```python
from build123d import *

# Parameters (mm, degrees)
CROQUIS1_W              = 4
CROQUIS1_H              = 15
CROQUIS1_W_2            = 15
CROQUIS1_W_3            = 16
CROQUIS1_R              = 1.5
SALIENTE_EXTRUIR1_DEPTH = 4
CROQUIS2_W              = 4
CROQUIS2_H              = 15
SALIENTE_EXTRUIR2_DEPTH = 60
SALIENTE_EXTRUIR4_START = -7.5
SALIENTE_EXTRUIR4_DEPTH = 15
CROQUIS8_R              = 2.85
CORTAR_EXTRUIR3_DEPTH   = 1.65
CORTAR_EXTRUIR2_REACH   = 114.965
CROQUIS7_R              = 1.5
CORTAR_EXTRUIR5_DEPTH   = 2
CROQUIS10_W             = 22
CROQUIS10_H             = 5
CORTAR_EXTRUIR6_DEPTH   = 22
CROQUIS11_W             = 13
CROQUIS11_H             = 14.4
SALIENTE_EXTRUIR5_DEPTH = 10


with BuildPart() as part:
    # Croquis1 → Saliente-Extruir1 (new body)
    # profile 1 of 3: a face of its own
    with BuildSketch(Plane.XY):
        with Locations((84, 80.273389683)):
            Rectangle(CROQUIS1_W, CROQUIS1_H)
    # profile 2 of 3: a face of its own
    with BuildSketch(Plane.XY):
        with Locations((74.5, 80.273389683)):
            Rectangle(CROQUIS1_W_2, CROQUIS1_H)
    # profile 3 of 3: a face of its own
    with BuildSketch(Plane.XY):
        with Locations((59, 80.273389683)):
            Rectangle(CROQUIS1_W_3, CROQUIS1_H)
        with Locations((55, 84.023389683)):
            Circle(CROQUIS1_R, mode=Mode.SUBTRACT)
        with Locations((63, 84.023389683)):
            Circle(CROQUIS1_R, mode=Mode.SUBTRACT)
    extrude(amount=SALIENTE_EXTRUIR1_DEPTH)

    # Croquis2 → Saliente-Extruir2 (add)
    with BuildSketch(Plane.XY.offset(4)):
        with Locations((84, 80.273389683)):
            Rectangle(CROQUIS2_W, CROQUIS2_H)
    extrude(amount=SALIENTE_EXTRUIR2_DEPTH)

    # Croquis6 → Saliente-Extruir4 (add)
    with BuildSketch(Plane(origin=(0, 80.273389683, 0), x_dir=(-1, 0, 0), z_dir=(0, -1, 0)).offset(SALIENTE_EXTRUIR4_START)):
        Polygon((-82, -30), (-82, -4), (-67, -4), align=None)
    extrude(amount=SALIENTE_EXTRUIR4_DEPTH)

    # Croquis8 → Cortar-Extruir3 (cut)
    with BuildSketch(Plane.XY.offset(4)):
        with Locations((63, 84.023389683)):
            Circle(CROQUIS8_R)
        with Locations((55, 84.023389683)):
            Circle(CROQUIS8_R)
    extrude(amount=-CORTAR_EXTRUIR3_DEPTH, mode=Mode.SUBTRACT)

    # Croquis7 → Cortar-Extruir2 (cut, up to next)
    with BuildSketch(Plane.ZY.offset(-82), mode=Mode.PRIVATE) as cortar_extruir2_sk1:
        with Locations((52.48, 76.973389683)):
            Circle(CROQUIS7_R)
    cortar_extruir2_tool1 = extrude(cortar_extruir2_sk1.sketch, amount=-CORTAR_EXTRUIR2_REACH, mode=Mode.PRIVATE) & part.part
    # Croquis7 → Cortar-Extruir2 (cut, up to next)
    with BuildSketch(Plane.ZY.offset(-82), mode=Mode.PRIVATE) as cortar_extruir2_sk2:
        with Locations((59.52, 83.573389683)):
            Circle(CROQUIS7_R)
    cortar_extruir2_tool2 = extrude(cortar_extruir2_sk2.sketch, amount=-CORTAR_EXTRUIR2_REACH, mode=Mode.PRIVATE) & part.part
    add(cortar_extruir2_tool1.solids().sort_by_distance((82, 76.97339, 52.48))[0], mode=Mode.SUBTRACT)
    add(cortar_extruir2_tool2.solids().sort_by_distance((82, 83.57339, 59.52))[0], mode=Mode.SUBTRACT)

    # Croquis9 → Cortar-Extruir5 (cut)
    with BuildSketch(Plane(origin=(86, 0, 0), x_dir=(0, 0, -1), z_dir=(1, 0, 0))):
        Polygon((-55.23, 75.385676443), (-52.48, 73.797963203), (-49.73, 75.385676443), (-49.73, 78.561102924), (-52.48, 80.148816164), (-55.23, 78.561102924), align=None)
        Polygon((-62.27, 81.985676443), (-59.52, 80.397963203), (-56.77, 81.985676443), (-56.77, 85.161102924), (-59.52, 86.748816164), (-62.27, 85.161102924), align=None)
    extrude(amount=-CORTAR_EXTRUIR5_DEPTH, mode=Mode.SUBTRACT)

    # Croquis10 → Cortar-Extruir6 (cut)
    with BuildSketch(Plane.ZY.offset(-51)):
        with Locations((11, 75.273389683)):
            Rectangle(CROQUIS10_W, CROQUIS10_H)
    extrude(amount=-CORTAR_EXTRUIR6_DEPTH, mode=Mode.SUBTRACT)

    # Croquis11 → Saliente-Extruir5 (add)
    with BuildSketch(Plane.XZ.offset(-72.773389683)):
        with Locations((79.5, 7.2)):
            Rectangle(CROQUIS11_W, CROQUIS11_H)
    extrude(amount=SALIENTE_EXTRUIR5_DEPTH)


solid = part.part
```
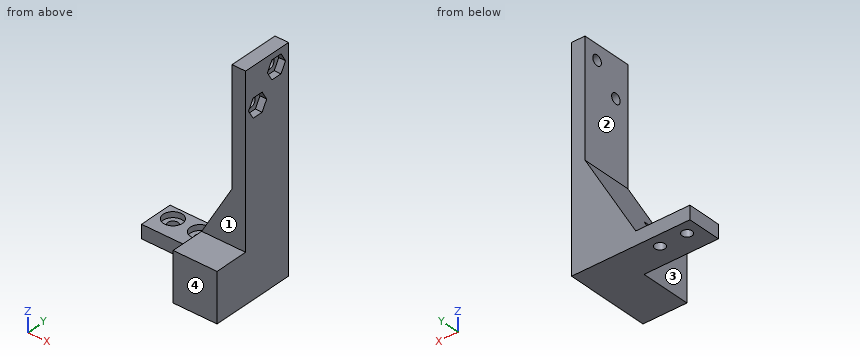
Part model, mm, in its own coordinate system. Face numbers are marked on the shaded views. A direction names the side the tool comes from. Round coordinates to 2 decimals unless told otherwise and drop trailing zeros. Loops run counter-clockwise (first coordinate to the right, second up) from the corner with the lowest first, then second, coordinate; pieces in that order, holes last.
Item 1: Drill centre lines: line 1 (Y direction, x = 63, z = 2); line 2 (Z direction, x = 85, y = 82); line 3 (Y direction, x = 63, z = 3.05). Where is each one in solid material? Low to high.
Item 2: Cut at C-C, the plane z = 10. Give the cut face in (x, y), then the cut area to 3 significant figures.
Item 3: Drop flat-ended pins along their axis: P1, Ø0.6, axis at x = 84.5, y = 84, coming from the -Z side; P2, Ø5, axis at x = 80, y = 67.5, coming from the +Z side; P3, Ø4.5, axis at x = 62, y = 85, coming from the +Z side; P4, Ø16, axis at x = 64.5, z = 6, coming from the -Y side. Give the stop position or say it passes through.
Item 4: Cut at B-B, the plane y = 69. Give the cut face in (x, z), then the cut area to 3 significant figures.
Item 5: Cut at A-A, the plane x = 55. Give the cut face in (y, z), then the cut area to 3 significant figures.
Item 6: 3-axis set-ups, long thin cutter, end or side, ignore diameter. For the marked faces 1, 2, 3 and 4: which of +Z, -Z, +X, -X, +Y, -Y reach the whole face in a straight line?
Item 7: Cut at D-D, the plane x = 78. Give the cut face in (y, z).
A:
1. line 1: y = 77.77 to 82.52, 85.52 to 87.77
1. line 2: z = 0 to 56.77, 62.27 to 64
1. line 3: y = 77.77 to 81.17, 86.87 to 87.77
2. outline: (70.46, 77.77) - (73, 77.77) - (73, 62.77) - (86, 62.77) - (86, 87.77) - (70.46, 87.77) - close
2. area: 350 mm2
3. P1: stops at z = 0
3. P2: stops at z = 14.4
3. P3: stops at z = 4
3. P4: stops at y = 77.77
4. outline: (73, 0) - (86, 0) - (86, 14.4) - (73, 14.4) - close
4. area: 187 mm2
5. outline: (77.77, 0) - (82.52, 0) - (82.52, 2.35) - (81.17, 2.35) - (81.17, 4) - (77.77, 4) - close; (85.52, 0) - (87.77, 0) - (87.77, 4) - (86.87, 4) - (86.87, 2.35) - (85.52, 2.35) - close
5. area: 23.5 mm2
6. face 1: +Z, +X, -X, -Y
6. face 2: +Z, -X, +Y, -Y
6. face 3: +Z, -Z, -X, -Y
6. face 4: +Z, -Z, +X, -X, -Y
7. outline: (62.77, 0) - (87.77, 0) - (87.77, 23.07) - (72.77, 23.07) - (72.77, 14.4) - (62.77, 14.4) - close
